from build123d import *

# Parameters (mm, degrees)
F0_R     = 125
F0_R_2   = 50
F1_DEPTH = 3
F3_D     = 5


with BuildPart() as f1:
    # F0 (on Top) → F1 (new body)
    with BuildSketch(Plane.XY):
        Circle(F0_R)
        Circle(F0_R_2, mode=Mode.SUBTRACT)
    extrude(amount=F1_DEPTH)

    # F3 (through all)
    with Locations(Plane.XY.offset(3)):
        with Locations((0, 110), (95.262794, -55), (-95.262794, -55)):
            Hole(F3_D / 2)


solid = f1.part
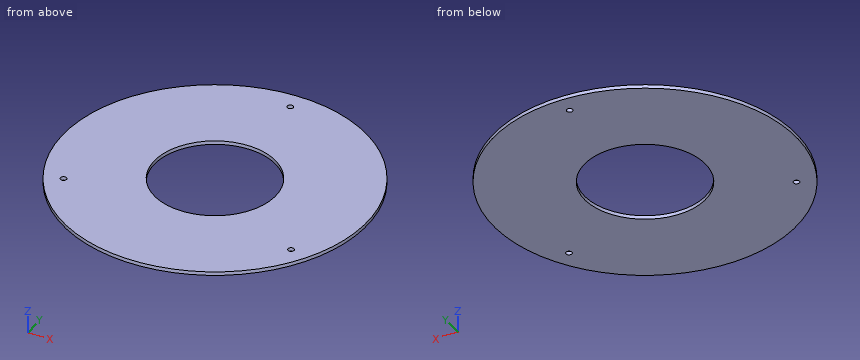
Could you check a few things on this model? Use its own coordinates, in mm. Give positions to 0.01 mm unless a question says otherwise; leave off trailing zeros. Order: outer loops, then holes, each group sorted by start corner. A loop starts at its lowest first (then second) coordinate and runs counter-clockwise, first axis right, second up. Notation, with made-up numbers: (7.25, -2.5) - (38.25, -2.5) arc R21 ccw to (38.25, 9.5) - close; hole circle Ø4 at (-21, 75.5). An arc over 180 degrees is marked (long way). Return JSON: item names as keys, results as strings. Group by question number.
Q1. Suppose I cut it at D-D, the plane x = -83.5. Please give me the cut outline in (y, z).
Q2. Suppose I cut it at A-A, the plane y = 0. Please give me the cut outline in (x, z).
Q3. Suppose I cut it at B-B, the plane z = 2.15. Please give me the cut outline in (x, y).
Q4. Will these pins go through, and if not, where does the flat tip stop? pin 1 Ø1.5 at (x, z) = (-92.5, 2.5) entering from +Y; pin 2 Ø1 at (x, z) = (32, 2) entering from +Y; pin 3 Ø1.5 at (y, z) = (56.5, 1) entering from +X.
Q5. Suppose I cut it at C-C, the plane x = -43. Please give me the cut outline in (y, z).
Q6. Please list where these lines run through material, in increasing order: line 1 along Y through (x, z) = (0, 0.85); line 2 along X through (y, z) = (-21.5, 1.6); line 3 along Y through (x, z) = (-34, 0.35). Write a range as [from, to].
Resolved:
{
 "1": {"outline": "(-93.02, 0) - (93.02, 0) - (93.02, 3) - (-93.02, 3) - close"},
 "2": {"outline": "(-125, 0) - (-50, 0) - (-50, 3) - (-125, 3) - close; (50, 0) - (125, 0) - (125, 3) - (50, 3) - close"},
 "3": {"outline": "circle Ø250 at (0, 0); hole circle Ø5 at (-95.26, -55); hole circle Ø100 at (0, 0); hole circle Ø5 at (0, 110); hole circle Ø5 at (95.26, -55)"},
 "4": {"pin 1": "stops at y = 84.89", "pin 2": "stops at y = 120.97", "pin 3": "stops at x = 111.88"},
 "5": {"outline": "(-117.37, 0) - (-25.51, 0) - (-25.51, 3) - (-117.37, 3) - close; (25.51, 0) - (117.37, 0) - (117.37, 3) - (25.51, 3) - close"},
 "6": {"line 1": "y = [-125, -50], [50, 107.5], [112.5, 125]", "line 2": "x = [-123.14, -45.14], [45.14, 123.14]", "line 3": "y = [-120.29, -36.66], [36.66, 120.29]"}
}
